Geometry: final body of the model. Coordinates: model frame, mm. A direction names the side the tool comes from. Give positions to 0.01 mm unless a question says otherwise; leave off trailing zeros. Write each loop counter-clockwise with the first axis right and the second up, starting at its lowest first coordinate (ties: lowest second). Pieces come first, ordered by that corner, then holes. Notation, with made-up numbers: (42, 9.5) - (90, 9.5) arc R18 cw to (90, 19.5) - close; hole circle Ø11 at (45, 46). An arc over 180 degrees is marked (long way). Use CSV: the item, a comma, the result in double quotes. Start each with the question number.
(1) Draft query along X for faces 1 (the cylindrical face through (4.38, -8.43, 8.98)), 2 (the flat face through (0, 10, 8.5)), 3 (the cylindrical face through (10, 3.2, 3.7)). Return one class per face: released by +X, released by -X, zero draft, split by the parting line, or undercut.
(2) Reachability of faces 4 (the flat face through (0, 0, 7.5)), 5 (the cylindrical face through (-2.54, -11.42, 4.19)) from +Z, -Z, +X, -X, +Y, -Y: full face, straight path, thin tool, end or side. Return the list, or none.
(3) First-contact query: pin 1 Ø3 at (y, z) = (-7, 9) entering from -X; pin 2 Ø6 at (x, y) = (-9, -8.5) entering from +Z; pin 3 Ø7 at (x, y) = (-4, 0.5) entering from +Z. Flat tips, straight axial feed; report the tip coordinate or a pass-through.
(4) Line query: probe 1 along X at (y, z) = (0.25, 3); probe 2 along Z at (x, y) = (-8.25, 7). Output: solid intervals per line, ascending. Write a range as [from, to].
(5) Section B-B on z = 10.25. Output: boundary loops of the cut face in (x, y), and give its area (3 significant figures).
(6) Section A-A on z = 3.75. Output: boundary loops of the cut face in (x, y).
from build123d import *

# Parameters (mm, degrees)
F0_R        = 11.7
F0_R_2      = 10.5
F1_DEPTH    = 8.5
F2_DEPTH    = 7.5
F3_R        = 9.5
F4_DEPTH    = 2
F7_T2_ANGLE = 180
F7_T4_ANGLE = 180


# Not quite as in the source:
# - a fillet or chamfer that OpenCascade refuses, or shapes differently, is made with other operations: its cross-section is extruded or revolved along the edge and cut away or added
# - a feature names something its author has since deleted; it is built from what else it names


with BuildPart() as f1:
    # F0 (on Top) → F1 (new body)
    with BuildSketch(Plane.XY):
        Circle(F0_R)
        Circle(F0_R_2, mode=Mode.SUBTRACT)
        Circle(F0_R_2)
    extrude(amount=F1_DEPTH)

    # F0 (on Top) → F2 (cut)
    with BuildSketch(Plane.XY):
        Circle(F0_R_2)
    extrude(amount=F2_DEPTH, mode=Mode.SUBTRACT)

    # F3 (on face) → F4 (join)
    with BuildSketch(Plane.XY.offset(8.5)):
        Circle(F3_R)
    extrude(amount=F4_DEPTH)

    # F5 (on Front) → F6 (revolve)
    with BuildSketch(Plane.XZ):
        with BuildLine():
            Line((-9.5, 10.5), (0, 10.5))
            Line((0, 10.5), (0, 13.5))
            ThreePointArc((0, 13.5), (-4.8754462608, 12.3972464927), (-9.5, 10.5))
        make_face()
    revolve(axis=Axis((0, 0, 12.3332124203), (0, 0, 1)))

    # F7: chamfer of 1 on 2 edges, made by hand

    # F7_s1 → F7_t2 (revolve, cut)
    with BuildSketch(Plane.XZ):
        with BuildLine():
            Line((-9.5214673898, 9.4467860572), (-8.5368878452, 10.9947550164))
            Line((-8.5368878452, 10.9947550164), (-8.5453666245, 11.0128688316))
            ThreePointArc((-8.5453666245, 11.0128688316), (-9.0246542065, 10.7600809063), (-9.5091067674, 10.5178063693))
            Line((-9.5091067674, 10.5178063693), (-9.52, 10.5))
            ThreePointArc((-9.52, 10.5), (-9.52, 9.9733930286), (-9.5414673898, 9.4467860572))
            Line((-9.5414673898, 9.4467860572), (-9.5214673898, 9.4467860572))
        make_face()
    revolve(axis=Axis((0, 0, 10.5), (0, 0, 1)), revolution_arc=F7_T2_ANGLE, mode=Mode.SUBTRACT)

    # F7_s3 → F7_t4 (revolve, cut)
    with BuildSketch(Plane.XZ):
        with BuildLine():
            Line((9.5214673898, 9.4467860572), (8.5368878452, 10.9947550164))
            Line((8.5368878452, 10.9947550164), (8.5453666245, 11.0128688316))
            ThreePointArc((8.5453666245, 11.0128688316), (9.0246542065, 10.7600809063), (9.5091067674, 10.5178063693))
            Line((9.5091067674, 10.5178063693), (9.52, 10.5))
            ThreePointArc((9.52, 10.5), (9.52, 9.9733930286), (9.5414673898, 9.4467860572))
            Line((9.5414673898, 9.4467860572), (9.5214673898, 9.4467860572))
        make_face()
    revolve(axis=Axis((0, 0, 10.5), (0, 0, 1)), revolution_arc=F7_T4_ANGLE, mode=Mode.SUBTRACT)


solid = f1.part
Check values:
1,face 1,"split by the parting line"
1,face 2,"zero draft"
1,face 3,"undercut"
2,face 4,"-Z"
2,face 5,"+Z, -Z"
3,pin 1,"stops at x = -10.28"
3,pin 2,"stops at z = 9.67"
3,pin 3,"stops at z = 13.42"
4,probe 1,"x = [-11.7, -10.5], [10.5, 11.7]"
4,probe 2,"z = [0, 8.5]"
5,outline,"circle Ø18.02 at (0, 0)"
5,area,"255 mm²"
6,outline,"circle Ø23.4 at (0, 0); hole circle Ø21 at (0, 0)"
